Could you check a few things on this model? Use its own coordinates, in mm. Face numbers are marked on the shaded views. A direction names the side the tool comes from. Round coordinates to 2 decimals unless told otherwise and drop trailing zeros. Order: outer loops, then holes, each group sorted by start corner. A loop starts at its lowest first (then second) coordinate and runs counter-clockwise, first axis right, second up.
```python
from build123d import *

# Parameters (mm, degrees)
SKETCH1_W                      = 20
SKETCH1_H                      = 20
BOSS_EXTRUDE1_DEPTH            = 2
BOSS_EXTRUDE3_DEPTH            = 1.5
SKETCH6_W                      = 4.75
SKETCH6_H                      = 20
BOSS_EXTRUDE4_DEPTH            = 3
TAP_DRILL_FOR_M2_2_HELICOIL1_D = 6.5


with BuildPart() as part:
    # Sketch1 → Boss-Extrude1 (new body)
    with BuildSketch(Plane(origin=(0, 0, 0), x_dir=(1, 0, 0), z_dir=(0, 1, 0))):
        Rectangle(SKETCH1_W, SKETCH1_H)
    extrude(amount=BOSS_EXTRUDE1_DEPTH)

    # Sketch3 → Boss-Extrude3 (add)
    with BuildSketch(Plane(origin=(0, 2, 0), x_dir=(1, 0, 0), z_dir=(0, 1, 0))):
        Polygon((-2.875, 8.25), (2.875, 8.25), (2.875, 2.867474963), (8.25, 2.867474963), (8.25, -2.882525037), (2.875, -2.875), (2.875, -8.25), (-2.875, -8.25), (-2.875, -2.875), (-8.25, -2.875), (-8.25, 2.875), (-2.875, 2.875), align=None)
    extrude(amount=BOSS_EXTRUDE3_DEPTH)

    # Sketch6 → Boss-Extrude4 (add)
    with BuildSketch(Plane.XZ):
        Rectangle(SKETCH6_W, SKETCH6_H)
    extrude(amount=BOSS_EXTRUDE4_DEPTH)

    # Tap Drill for M2.2 Helicoil1 (through all)
    with Locations(Plane.ZX.offset(3.5)):
        with Locations((0, 0)):
            Hole(TAP_DRILL_FOR_M2_2_HELICOIL1_D / 2)


solid = part.part
```
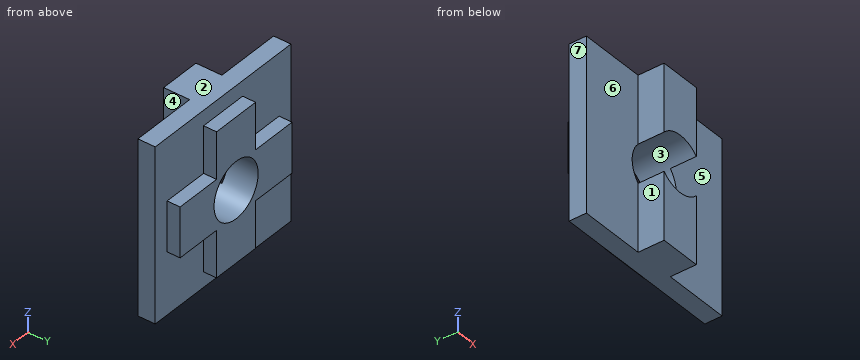
Q1. We'd pull the mould along X, two halves only. Please class the marked faces 1, 2, 3 and 4: released by +X, released by -X, zero draft, split by the parting line, or undercut.
Q2. Imagine slicing it at D-D, the plane y = 2.25. Please give me the cut outline in (x, z) (3 decimals), then the cut area to 3 significant figures.
Q3. I need wall thicknesses on L1, parallel to Z at x = 0, y = -0.5; L2, parallel to X at y = 2.25, z = 0; L3, parallel to Y at x = 7.75, z = -5. Which ranges of each line are inside material? Lowest first, please.
Q4. Imagine slicing it at B-B, the plane z = 0. Please give me the cut outline in (x, y), then the cut area to 3 significant figures.
Q5. Imagine slicing it at A-A, the plane x = 0. Please give me the cut outline in (y, z), then the cut area to 3 significant figures.
Q6. For the marked faces 5, 6 and 7, which set-ups out of +Z, -Z, +X, -X, +Y, -Y let a thin tool reach every point of the face, with its end or its side?
Q7. Imagine slicing it at C-C, the plane y = -1.25. Please give me the cut outline in (x, z) (3 decimals).
Q8. For P1, Ø0.8, axis at x = 0, y = 2.5, coming from the +Z side; P2, Ø1.5, axis at x = -3, z = -3.5, coming from the +Y side; P3, Ø1.2, axis at y = 3, z = 5, coming from the +X side (3 decimals); P4, Ø1.5, axis at y = -2, z = 0.5, coming from the +X side, each with a flat end and sliding along its axis, tell me the tip position at first contact or that it passes through.
Filled in:
1. face 1: released by -X
1. face 2: zero draft
1. face 3: undercut
1. face 4: released by +X
2. outline: (-8.25, -2.875) - (-2.875, -2.875) - (-2.875, -8.25) - (2.875, -8.25) - (2.875, -2.867) - (8.25, -2.867) - (8.25, 2.883) - (2.875, 2.875) - (2.875, 8.25) - (-2.875, 8.25) - (-2.875, 2.875) - (-8.25, 2.875) - close; hole circle Ø6.5 at (0, 0)
2. area: 123 mm2
3. L1: z = -10 to -3.25, 3.25 to 10
3. L2: x = -8.25 to -3.25, 3.25 to 8.25
3. L3: y = 0 to 2
4. outline: (-10, 0) - (-3.25, 0) - (-3.25, 3.5) - (-8.25, 3.5) - (-8.25, 2) - (-10, 2) - close; (3.25, 0) - (10, 0) - (10, 2) - (8.25, 2) - (8.25, 3.5) - (3.25, 3.5) - close
4. area: 42.0 mm2
5. outline: (-3, -10) - (2, -10) - (2, -8.25) - (3.5, -8.25) - (3.5, -3.25) - (-3, -3.25) - close; (-3, 3.25) - (3.5, 3.25) - (3.5, 8.25) - (2, 8.25) - (2, 10) - (-3, 10) - close
5. area: 82.5 mm2
6. face 5: +Z, -Z, +X, -Y
6. face 6: +Z, -Z, -X, -Y
6. face 7: +Z, -Z, -X, +Y, -Y
7. outline: (-2.375, -10) - (2.375, -10) - (2.375, -2.219) arc R3.25 cw to (-2.375, -2.219) - close; (-2.375, 2.219) arc R3.25 cw to (2.375, 2.219) - (2.375, 10) - (-2.375, 10) - close
8. P1: stops at z = 8.25
8. P2: stops at y = 3.5
8. P3: stops at x = 2.875
8. P4: passes through
